The listing builds one solid part. Answer for the finished solid, in the listing's coordinates (mm). A direction names the side the tool comes from. Coordinates: 2 decimals unless noted, no trailing zeros. Order: outer loops, then holes, each group sorted by start corner. A loop starts at its lowest first (then second) coordinate and runs counter-clockwise, first axis right, second up. Notation, with made-up numbers: (53.5, 65) -> (65.5, 65) arc R19 cw to (65.5, 85) -> close; hole circle Ø11 at (25, 81.5). An arc over 180 degrees is marked (long way). One line per question, with ' | ' between items.
from build123d import *
from OCP.BRepFilletAPI import BRepFilletAPI_MakeChamfer

# Parameters (mm, degrees)
CHAFL_N1_SIZE  = 3
CHAFL_N1_SIZE2 = 3.300188603
CHAFL_N2_SIZE  = 0.5


with BuildPart() as part:
    # Croquis1 → Revolución1 (revolve)
    with BuildSketch(Plane.XY, mode=Mode.PRIVATE) as revoluci_n1_sk:
        Polygon((114.5, 12.5), (98, 12.5), (98, 5), (157, 5), (157, 0), (239, 0), (239, 5), (298, 5), (298, 12.5), (281.5, 12.5), (278.219175118, 50), (117.780824882, 50), align=None)
    revolve(revoluci_n1_sk.sketch.rotate(Axis((26.636942393, 0, 0), (1, 0, 0)), 90), axis=Axis((26.636942393, 0, 0), (1, 0, 0)))

    # Chaflán1: one chamfer whose edges measure the first distance from different faces: ONE call of the kernel's chamfer builder (chamfer() names one face for all edges)
    chafl_n1_edges_1 = [part.edges().sort_by_distance(p)[0] for p in [
        (117.780824882, 0, -50),
    ]]
    chafl_n1_side_1 = [part.faces().sort_by_distance(p)[0] for p in [
        (198, 0, -50),
    ]]
    chafl_n1_edges_2 = [part.edges().sort_by_distance(p)[0] for p in [
        (278.219175118, 0, -50),
    ]]
    chafl_n1_side_2 = [part.faces().sort_by_distance(p)[0] for p in [
        (279.859587559, 0, -31.25),
    ]]
    chafl_n1 = BRepFilletAPI_MakeChamfer(part.part.solid().wrapped)
    for e in chafl_n1_edges_1:
        chafl_n1.Add(CHAFL_N1_SIZE, CHAFL_N1_SIZE2, e.wrapped, chafl_n1_side_1[0].wrapped)  # the first distance lies on this face
    for e in chafl_n1_edges_2:
        chafl_n1.Add(CHAFL_N1_SIZE, CHAFL_N1_SIZE2, e.wrapped, chafl_n1_side_2[0].wrapped)  # the first distance lies on this face
    add(Compound.cast(chafl_n1.Shape()), mode=Mode.REPLACE)

    # Chaflán2
    chafl_n2_edges = [part.edges().sort_by_distance(p)[0] for p in [
        (298, 0, -12.5),
        (98, 0, -12.5),
    ]]
    chamfer(chafl_n2_edges, length=CHAFL_N2_SIZE)


solid = part.part
Item 1: Find the intervals of material crossed by L1, parallel to Y at x = 110, z = 0; L2, parallel to Y at x = 271, z = 0; L3, parallel to X at y = 12.5, z = 45, in increasing order.
Computed values:
L1: y = -12.5 to -5, 5 to 12.5 | L2: y = -50 to -5, 5 to 50 | L3: x = 117.49 to 278.51
Item 2: Each of these flat-tipped pins is pushed along its axis until it touches: pin 1 Ø5 at (x, y) = (255.5, -12) entering from +Z; pin 2 Ø1 at (x, y) = (158, 2.5) entering from -Z; pin 3 Ø4 at (x, y) = (229, 23) entering from +Z. Where does it stop, or does it pass through?
Computed values:
pin 1: stops at z = 49.09 | pin 2: stops at z = -49.96 | pin 3: stops at z = 45.38
Item 3: Determine the mould class of faces 4 (the face through (157, 0, 0)), 5 (the face through (106.388, -3.755, 11.923)), 6 (the face through (239, 0, 0)), 7 (the face through (298, -0.2, -5.2)) for opening direction Z: pulls with the +Z half, pulls with the -Z half, needs draft (parallel to the pull), parting line crosses it, or undercut.
Computed values:
face 4: undercut | face 5: parting line crosses it | face 6: undercut | face 7: needs draft
Item 4: Section B-B, the plane x = 211 is taken. Give the vertices of the cut face in (y, z), plus the area to 3 significant figures.
Computed values:
outline: circle Ø100 at (0, 0) | area: 7,850 mm^2
Item 5: Section A-A, the plane x = 147 is taken. Give the vertices of the cut face in (y, z).
Computed values:
outline: circle Ø100 at (0, 0); hole circle Ø10 at (0, 0)
Item 6: For faces 1 (the face through (128, 0, -5)), 2 (the face through (98, -0.2, 5.2)), 3 (the face through (289.388, -3.755, 11.923)), determine the directions among +Z, -Z, +X, -X, +Y, -Y from which every point of the face is accessible in a straight line to the end or side of a thin tool.
Computed values:
face 1: -X | face 2: +Z, -Z, -X, +Y, -Y | face 3: +X
